Read the model definition and answer for the solid it produces. Units are mm, in the model's axes. Coordinates: 2 decimals unless noted, no trailing zeros. Write each loop counter-clockwise with the first axis right and the second up, starting at its lowest first coordinate (ties: lowest second). Pieces come first, ordered by that corner, then holes. Notation, with made-up numbers: (-11.75, -14.75) -> (-1.75, -14.75) arc R25 cw to (-1.75, 6.25) -> close; hole circle Ø5 at (15.5, 39). An arc over 180 degrees is marked (long way). Answer in a Markdown table with one row per item. Add a question column.
Item 1: Section D-D on x = -6 is taken. Write down the section's boundary in (y, z), then the cut area to 3 significant figures.
Item 2: Section C-C on x = 2.25 is taken. Write down the section's boundary in (y, z), then the cut area to 3 significant figures.
Item 3: For a pull along X with two mould halves and no side action, classify faces 1 (the face through (10.977, 0.986, -0.248)), 2 (the face through (-11.09, 0.99, -0.02)), 3 (the face through (0, 0, 0)), 4 (the face through (-9.665, 0.986, -0.165)) as +X half, -X half, draft (parallel to the pull), parting line (faces both ways), or undercut.
Item 4: Section A-A on z = 0 is taken. Write down the section's boundary in (x, y) (3 decimals).
Item 5: Straight lines are drawn through the part: line 1 (X direction, y = 1.7, z = 0.05); line 2 (Z direction, x = -10.19, y = 1.5); line 3 (X direction, y = 1, z = -0.15). For each, find the intervals that lie inside material, in ascending order. Write a range as from..to.
Item 6: Section B-B on y = 0.95 is taken. Write down the section's boundary in (x, z) (3 decimals).
```python
from build123d import *

# Parameters (mm, degrees)
SKETCH1_R           = 0.55
SKETCH1_R_2         = 0.825
BOSS_EXTRUDE1_DEPTH = 2


with BuildPart() as part:
    # Sketch1 → Boss-Extrude1 (new body)
    with BuildSketch(Plane(origin=(0, 0, 0), x_dir=(1, 0, 0), z_dir=(0, 1, 0))):
        with BuildLine():
            Line((10.14707841, 1.249262877), (-10.19, 0.9))
            ThreePointArc((-10.19, 0.9), (-11.09, 0), (-10.19, -0.9))
            Line((-10.19, -0.9), (10.14707841, -1.249262877))
            Line((10.14707841, -1.249262877), (10.19, -1.25))
            ThreePointArc((10.19, -1.25), (11.44, 0), (10.19, 1.25))
            Line((10.19, 1.25), (10.14707841, 1.249262877))
        make_face()
        with Locations((-10.19, 0)):
            Circle(SKETCH1_R, mode=Mode.SUBTRACT)
        with Locations((10.19, 0)):
            Circle(SKETCH1_R_2, mode=Mode.SUBTRACT)
    extrude(amount=BOSS_EXTRUDE1_DEPTH)


solid = part.part
```
Results below:
| question | item | result |
|---|---|---|
| 1 | outline | (0, -0.97) -> (2, -0.97) -> (2, 0.97) -> (0, 0.97) -> close |
| 1 | area | 3.89 mm2 |
| 2 | outline | (0, -1.11) -> (2, -1.11) -> (2, 1.11) -> (0, 1.11) -> close |
| 2 | area | 4.45 mm2 |
| 3 | face 1 | undercut |
| 3 | face 2 | -X half |
| 3 | face 3 | draft |
| 3 | face 4 | undercut |
| 4 | outline | (-11.09, 0) -> (-10.74, 0) -> (-10.74, 2) -> (-11.09, 2) -> close; (-9.64, 0) -> (9.365, 0) -> (9.365, 2) -> (-9.64, 2) -> close; (11.015, 0) -> (11.44, 0) -> (11.44, 2) -> (11.015, 2) -> close |
| 5 | line 1 | x = -11.09..-10.74, -9.64..9.37, 11.01..11.44 |
| 5 | line 2 | z = -0.9..-0.55, 0.55..0.9 |
| 5 | line 3 | x = -11.08..-10.72, -9.66..9.38, 11..11.43 |
| 6 | outline | (-10.19, -0.9) -> (10.19, -1.25) arc R1.25 ccw to (10.19, 1.25) -> (-10.19, 0.9) arc R0.9 ccw to start; hole circle Ø1.1 at (-10.19, 0); hole circle Ø1.65 at (10.19, 0) |
